Autodesk Inventor part; units mm, degrees
ref_plane "YZ Plane" through (0, 0, 0) normal (1, 0, 0) x (0, 1, 0)
ref_plane "XZ Plane" through (0, 0, 0) normal (0, 1, 0) x (-1, 0, 0)
ref_plane "XY Plane" through (0, 0, 0) normal (0, 0, 1) x (1, 0, 0)
sketch "Sketch1" plane through (0, 0, 0) normal (0, 0, 1) x (1, 0, 0)
  circle A0 centre (0, 0) radius 4.825
  dimension "d0" = 9.65
extrude "Extrusion1" add sketch "Sketch1" along normal blind 85
chamfer "Chamfer1" distance 1 angle 45 2 edges at (-4.825, 0, 85) (-4.825, 0, 0)
sketch "Sketch2" plane through (0, 0, 0) normal (0, 1, 0) x (-1, 0, 0)
  line L0 (4.825, 1) -> (4.825, 84)
  line L1 (4.825, 1.69) -> (4.325, 1.69)
  line L2 (4.325, 1.69) -> (4.325, 2.67)
  line L3 (4.325, 2.67) -> (4.825, 2.67)
  line L4 (4.825, 2.67) -> (4.825, 1.69)
  line L5 (0, -17) -> (0, 102)
  point P0 (0, 0)
  dimension "d6" = 0.5
  dimension "d7" = 0.98
  dimension "d8" = 0.69
revolve "Revolution1" cut sketch "Sketch2" angle 360 about axis through (0, 0, -10) along (0, 0, 1)
properties part number "Shaft"
Source: CAD feature listing. Evaluate the final solid. Frame: model axes, mm. Give positions to 0.01 mm unless a question says otherwise; leave off trailing zeros. Write each loop counter-clockwise with the first axis right and the second up, starting at its lowest first coordinate (ties: lowest second). Pieces come first, ordered by that corner, then holes. Notation, with made-up numbers: M 13.5,26 L 19.5,26 A21 ccw 19.5,31 Z; hole C 85,76.5 d4. An arc over 180 degrees is marked long. Return JSON: item names as keys, results as strings. Group by question number.
1) Cut plane A-A, the plane z = 23. Output: boundary loops of the cut face in (x, y) (3 decimals).
2) Pull-direction query (Z, two-part tool) for faces 1 (the face through (-4.125, -1.299, 2.187)), 2 (the face through (4.6, -1.45, 42.77)), 3 (the face through (0, 0, 85)), 4 (the face through (0, 0, 0)); classes: pulls with the +Z half, pulls with the -Z half, needs draft (parallel to the pull), parting line crosses it, or undercut.
3) Material intervals for line 1 along Z through (x, y) = (3.75, 2.5); line 2 along X through (y, z) = (0.25, 56); line 3 along X through (y, z) = (-2.25, 19.5), sorted ascending. Write a range as [from, to].
4) Pin query (flat end, axial travel): P1, Ø4, axis at y = 3.5, z = 37.5, coming from the +X side; P2, Ø5, axis at y = 2.5, z = 60.5, coming from the -X side (3 decimals); P3, Ø5, axis at x = 3.5, z = 8.5, coming from the -Y side; P4, Ø1.5, axis at y = -2.5, z = 51, coming from the +X side. Return the tip coordinate at first contact, or that it passes through.
Recorded:
{
 "1": {"outline": "C 0,0 d9.65"},
 "2": {"face 1": "undercut", "face 2": "needs draft", "face 3": "pulls with the +Z half", "face 4": "pulls with the -Z half"},
 "3": {"line 1": "z = [0.68, 1.69], [2.67, 84.32]", "line 2": "x = [-4.82, 4.82]", "line 3": "x = [-4.27, 4.27]"},
 "4": {"P1": "stops at x = 4.59", "P2": "stops at x = -4.825", "P3": "stops at y = -4.72", "P4": "stops at x = 4.5"}
}
